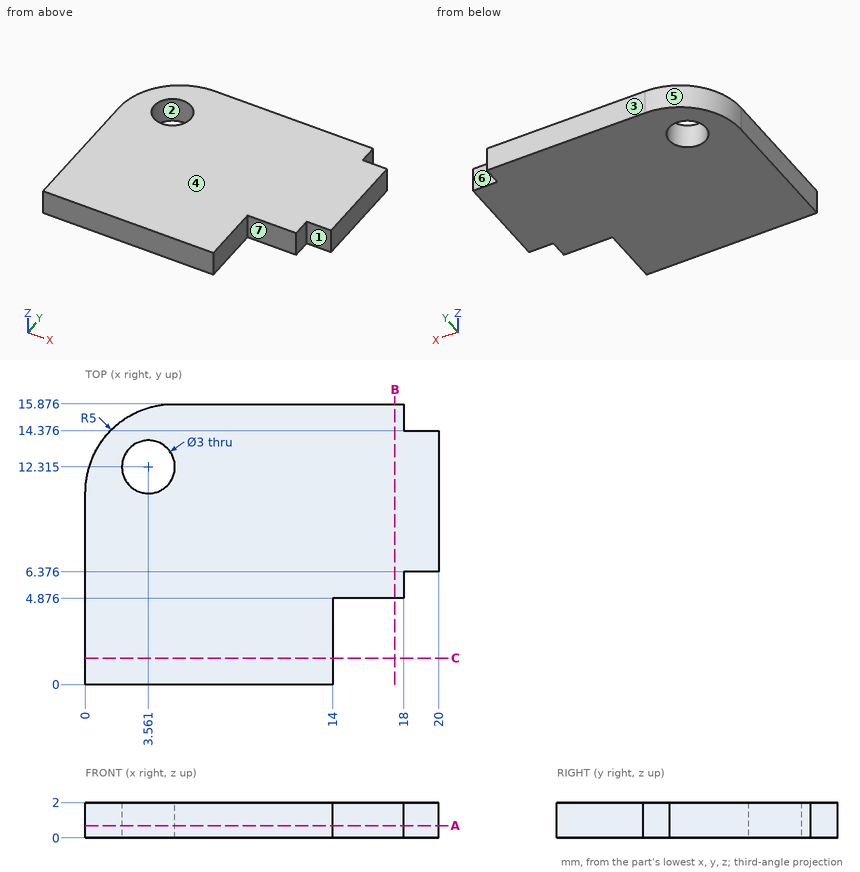
The figure shows three views and two pictorial views of one solid part (mm, origin at its lowest corner). Answer the questions. A direction names the side the tool comes from. Round coordinates to 2 decimals unless told otherwise and drop trailing zeros. Order: outer loops, then holes, each group sorted by start corner. A loop starts at its lowest first (then second) coordinate and runs counter-clockwise, first axis right, second up.
Q1. Find the intervals of material crossed by line 1 along Y through (x, z) = (18.5, 0.7) (1 decimal); line 2 along Y through (x, z) = (16.5, 1.15) (1 decimal); line 3 along X through (y, z) = (6.25, 1.2), in increasing order.
Solution:
line 1: y = 6.4 to 14.4
line 2: y = 4.9 to 15.9
line 3: x = 0 to 18
Q2. A tool of negligible diameter and unlimited length cuts with its end or side. For the marked faces 5, 6 and 7, from which of +Z, -Z, +X, -X, +Y, -Y can it reach the whole face along a straight path? Write none if from no direction.
Solution:
face 5: +Z, -Z, -X, +Y
face 6: +Z, -Z, +X, +Y
face 7: +Z, -Z, +X, -Y
Q3. A cutting plane is placed at C-C, the plane y = 1.5. Determine the outline of the cut face in (x, z), then the cut area to 3 significant figures.
Solution:
outline: (0, 0) - (14, 0) - (14, 2) - (0, 2) - close
area: 28.0 mm2
Q4. Given pin 1 Ø1 at (x, z) = (17, 0.5) entering from -Y; pin 2 Ø0.8 at (y, z) = (5.5, 1.5) entering from +X, each flat-ended and moving along its own axis, determine where each tip first touches the part or whether it passes through.
Solution:
pin 1: stops at y = 4.88
pin 2: stops at x = 18
Q5. The mould has two halves that part along Y. Classify the marked faces 1, 2, 3 and 4: pulls with the +Y half, pulls with the -Y half, needs draft (parallel to the pull), parting line crosses it, or undercut.
Solution:
face 1: pulls with the -Y half
face 2: undercut
face 3: pulls with the +Y half
face 4: needs draft
Q6. A cutting plane is placed at A-A, the plane z = 0.7. Determine the outline of the cut face in (x, y) (1 decimal), then the cut area to 3 significant figures.
Solution:
outline: (0, 0) - (14, 0) - (14, 4.9) - (18, 4.9) - (18, 6.4) - (20, 6.4) - (20, 14.4) - (18, 14.4) - (18, 15.9) - (5, 15.9) arc R5 ccw to (0, 10.9) - close; hole circle Ø3 at (3.6, 12.3)
area: 270 mm2
Q7. A cutting plane is placed at B-B, the plane x = 17.5. Determine the outline of the cut face in (y, z) (1 decimal).
Solution:
outline: (4.9, 0) - (15.9, 0) - (15.9, 2) - (4.9, 2) - close
